Work out the finished part from the listing and answer in its coordinate system (mm). A direction names the side the tool comes from. Give positions to 0.01 mm unless a question says otherwise; leave off trailing zeros. Write each loop counter-clockwise with the first axis right and the second up, starting at its lowest first coordinate (ties: lowest second). Pieces come first, ordered by that corner, then holes.
1) Given pin 1 Ø2.5 at (y, z) = (-31.5, 3.5) entering from +X; pin 2 Ø2.5 at (y, z) = (-100, 3.5) entering from -X, each flat-ended and moving along its own axis, determine where each tip first touches the part or whether it passes through.
2) Find section A-A (z = 1.2). Determine the outline of the cut face in (x, y).
3) Straight lines are drawn through the part: probe 1 along X at (y, z) = (-18.5, 0.9); probe 2 along Y at (x, z) = (33, 1.4); probe 3 along Y at (x, z) = (15.5, 1.1). For each, find the intervals that lie inside material, in ascending order.
4) Find section C-C (x = 40). Determine the outline of the cut face in (y, z), plus the area to 3 significant figures.
5) Find section B-B (y = -79). Determine the outline of the cut face in (x, z), plus the area to 3 significant figures.
6) A tool of negligible diameter and unlimited length cuts with its end or side. For faces 1 (the face through (69, -98, 2)), 2 (the face through (31, -86.5, 2)), from which of +Z, -Z, +X, -X, +Y, -Y can it reach the whole face along a straight path? Write none if from no direction.
```python
from build123d import *

# Parameters (mm, degrees)
BOSS_EXTRUDE1_DEPTH = 5
SKETCH2_W           = 0.1
SKETCH2_H           = 5
CUT_EXTRUDE2_DEPTH  = 3


with BuildPart() as part:
    # Sketch1 → Boss-Extrude1 (new body)
    with BuildSketch(Plane.XY):
        with BuildLine():
            Line((0, -1), (0, -96.5))
            ThreePointArc((0, -96.5), (1.464466094, -100.035533906), (5, -101.5))
            Line((5, -101.5), (68, -101.5))
            ThreePointArc((68, -101.5), (68.707106781, -101.207106781), (69, -100.5))
            Line((69, -100.5), (69, -96.429996046))
            ThreePointArc((69, -96.429996046), (68.042547906, -93.487580979), (65.53687743, -91.672054499))
            Line((65.53687743, -91.672054499), (57.01873992, -88.920584529))
            ThreePointArc((57.01873992, -88.920584529), (49.429079532, -87.108853154), (41.649965621, -86.5))
            Line((41.649965621, -86.5), (20, -86.5))
            ThreePointArc((20, -86.5), (16.464466094, -85.035533906), (15, -81.5))
            Line((15, -81.5), (15, -61))
            Line((15, -61), (15, 0))
            Line((15, 0), (0, 0))
            Line((0, 0), (0, -1))
        make_face()
    extrude(amount=BOSS_EXTRUDE1_DEPTH)

    # Sketch2 → Cut-Extrude2 (cut)
    with BuildSketch(Plane.XZ.offset(101.5)):
        with Locations((64.9, 2.5)):
            Rectangle(SKETCH2_W, SKETCH2_H)
    extrude(amount=-CUT_EXTRUDE2_DEPTH, mode=Mode.SUBTRACT)


solid = part.part
```
Results:
1. pin 1: stops at x = 15
1. pin 2: stops at x = 0.53
2. outline: (0, -96.5) arc R5 ccw to (5, -101.5) - (64.85, -101.5) - (64.85, -98.5) - (64.95, -98.5) - (64.95, -101.5) - (68, -101.5) arc R1 ccw to (69, -100.5) - (69, -96.43) arc R5 ccw to (65.54, -91.67) - (57.02, -88.92) arc R50 ccw to (41.65, -86.5) - (20, -86.5) arc R5 cw to (15, -81.5) - (15, 0) - (0, 0) - close
3. probe 1: x = 0 to 15
3. probe 2: y = -101.5 to -86.5
3. probe 3: y = -101.5 to -83.68
4. outline: (-101.5, 0) - (-86.5, 0) - (-86.5, 5) - (-101.5, 5) - close
4. area: 75.0 mm2
5. outline: (0, 0) - (15, 0) - (15, 5) - (0, 5) - close
5. area: 75.0 mm2
6. face 1: +Z, -Z, +X, +Y, -Y
6. face 2: +Z, -Z, +X, +Y
